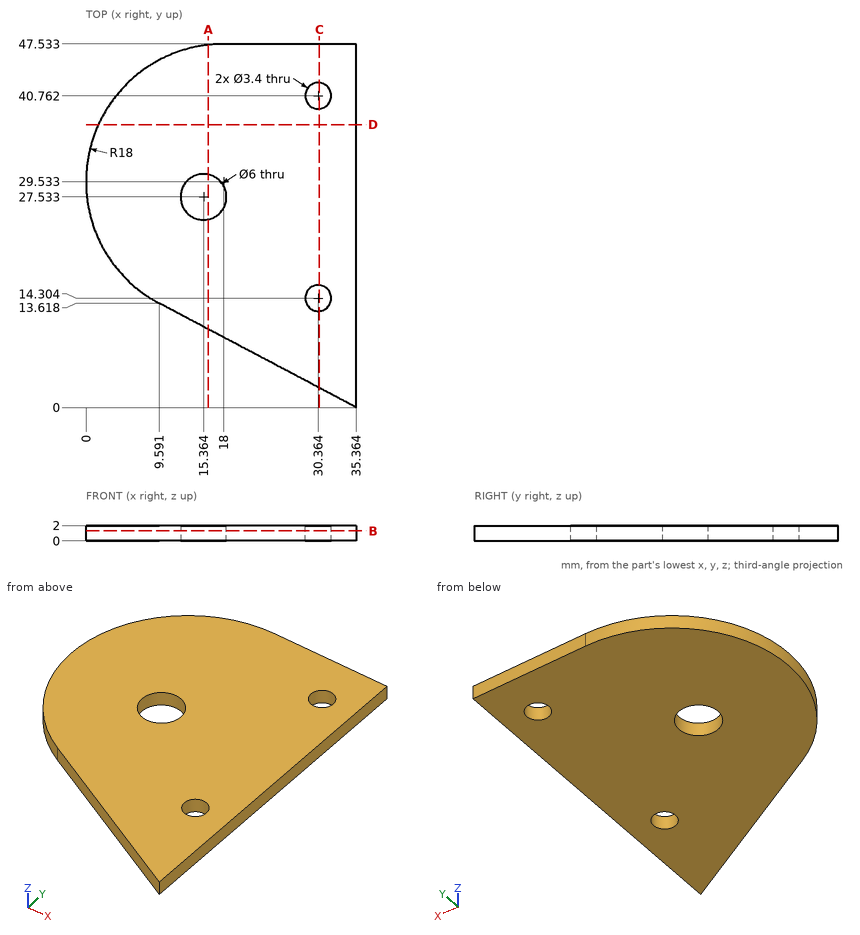
Here's the drawing with two shaded views (mm, measured from the low corner). I have some questions. Coordinates: 2 decimals unless noted, no trailing zeros. Order: outer loops, then holes, each group sorted by start corner. A loop starts at its lowest first (then second) coordinate and runs counter-clockwise, first axis right, second up. Notation, with made-up numbers: (75.25, 89.5) - (109.25, 89.5) arc R21 cw to (109.25, 108.5) - close; hole circle Ø5 at (20.25, 31.5). An arc over 180 degrees is marked (long way). Answer in a Markdown table with one row per item. Add a question column.
(1) If we section it at C-C, the plane x = 30.5: Please give me the cut outline in (y, z).
(2) If we section it at A-A, the plane x = 16: Please give me the cut outline in (y, z) (1 decimal).
(3) If we section it at B-B, the plane z = 1.3: Please give me the cut outline in (x, y).
(4) Will this pin go through, and if not, where does the flat tip stop? pin 1 (3.5 mm diameter, centred on x = 15.36, y = 27.53, fed in from +Z).
(5) If we section it at D-D, the plane y = 37: Please give me the cut outline in (x, z).
(6) I need wall thicknesses on L1, parallel to X at y = 15, z = 0.4 (1 decimal); L2, parallel to Y at x = 13, z = 0.45 (1 decimal); L3, parallel to X at y = 27.5, z = 0.75 (1 decimal). Which ranges of each line are inside material? Lowest first, please.
Results are:
| question | item | result |
|---|---|---|
| 1 | outline | (2.57, 0) - (12.61, 0) - (12.61, 2) - (2.57, 2) - close; (16, 0) - (39.07, 0) - (39.07, 2) - (16, 2) - close; (42.46, 0) - (47.53, 0) - (47.53, 2) - (42.46, 2) - close |
| 2 | outline | (10.2, 0) - (24.6, 0) - (24.6, 2) - (10.2, 2) - close; (30.5, 0) - (47.4, 0) - (47.4, 2) - (30.5, 2) - close |
| 3 | outline | (9.59, 13.62) - (35.36, 0) - (35.36, 47.53) - (18, 47.53) arc R18 ccw to start; hole circle Ø6 at (15.36, 27.53); hole circle Ø3.4 at (30.36, 14.3); hole circle Ø3.4 at (30.36, 40.76) |
| 4 | pin 1 | passes through |
| 5 | outline | (1.62, 0) - (35.36, 0) - (35.36, 2) - (1.62, 2) - close |
| 6 | L1 | x = 7.4 to 28.8, 31.9 to 35.4 |
| 6 | L2 | y = 11.8 to 25.7, 29.4 to 46.8 |
| 6 | L3 | x = 0.1 to 12.4, 18.4 to 35.4 |
